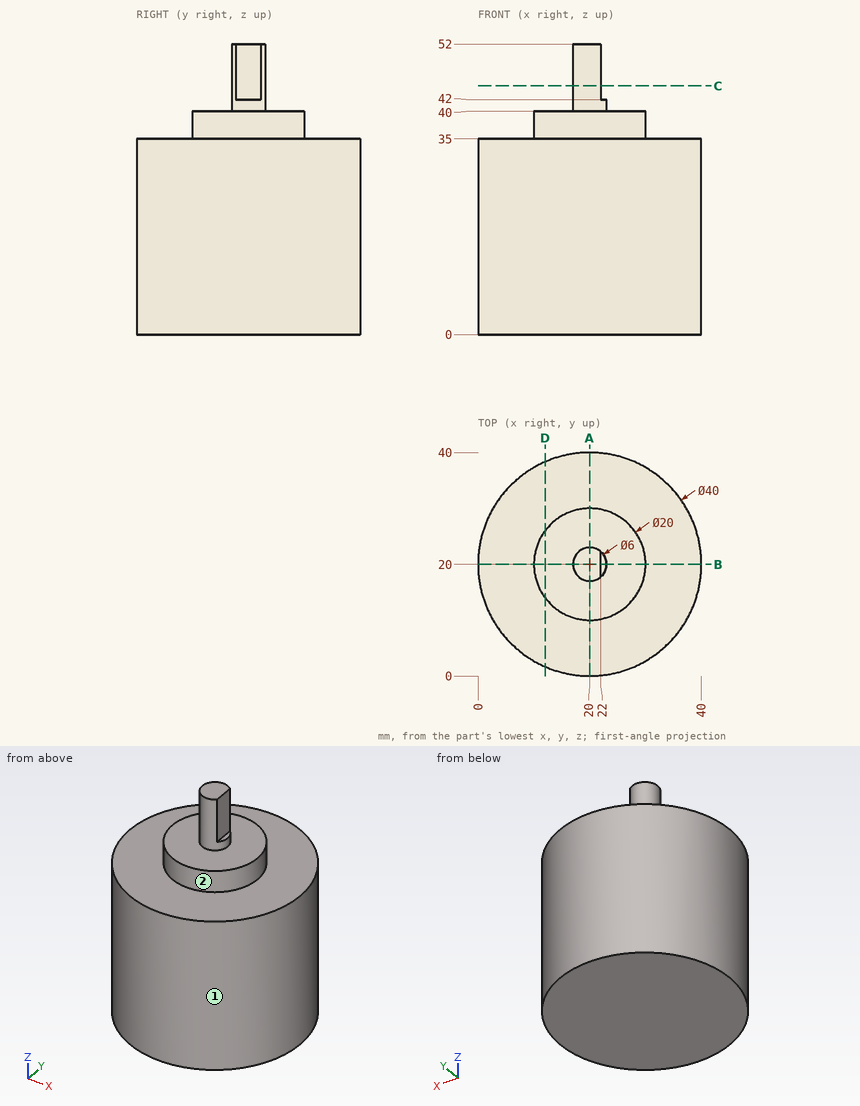
Verification items for this drawing (mm, ordinates from the low corner). A direction names the side the tool comes from. Round coordinates to 2 decimals unless told otherwise and drop trailing zeros. Loops run counter-clockwise (first coordinate to the right, second up) from the corner with the lowest first, then second, coordinate; pieces in that order, holes last. Notation, with made-up numbers: M -6.5,89 L 12.5,89 A18 cw 12.5,113 Z; hole C 73.25,89.5 d9. An arc over 180 degrees is marked long. Answer as a JSON object with one key per item and string values.
1. Section check B-B (y = 20). Record the boundary of the cut face in (x, z), plus the area to 3 significant figures.
Reply:
{"outline": "M 0,0 L 40,0 L 40,35 L 30,35 L 30,40 L 23,40 L 23,42 L 22,42 L 22,52 L 17,52 L 17,40 L 10,40 L 10,35 L 0,35 Z", "area": "1,560 mm²"}
2. Gauge pin test, flat ends, axial feed: P1, Ø10, axis at y = 14.5, z = 29.5, coming from the -X side; P2, Ø0.5, axis at x = 22.5, y = 19, coming from the +Z side; P3, Ø6, axis at x = 17, z = 45.5, coming from the +Y side. Record the tip position at first contact, or that the pin passes through.
Reply:
{"P1": "stops at x = 0.01", "P2": "stops at z = 42", "P3": "stops at y = 23"}
3. Section check A-A (x = 20). Record the boundary of the cut face in (y, z).
Reply:
{"outline": "M 0,0 L 40,0 L 40,35 L 30,35 L 30,40 L 23,40 L 23,52 L 17,52 L 17,40 L 10,40 L 10,35 L 0,35 Z"}
4. Scan lines: line 1 (Z direction, x = 33, y = 28); line 2 (Z direction, x = 20, y = 11.5); line 3 (X direction, y = 34, z = 27). Record each from-to range of solid material in increasing order.
Reply:
{"line 1": "z = 0 to 35", "line 2": "z = 0 to 40", "line 3": "x = 5.72 to 34.28"}
5. Section check D-D (x = 12). Record the boundary of the cut face in (y, z).
Reply:
{"outline": "M 1.67,0 L 38.33,0 L 38.33,35 L 26,35 L 26,40 L 14,40 L 14,35 L 1.67,35 Z"}
6. Section check C-C (z = 44.5). Record the boundary of the cut face in (x, y), plus the area to 3 significant figures.
Reply:
{"outline": "M 22,17.76 L 22,22.24 A3 ccw long Z", "area": "25.2 mm²"}
7. Access from +Z, -Z, +X, -X, +Y, -Y to the whole of each face (thin tool, end or side, straight path). Record for the marked faces 1 and 2.
Reply:
{"face 1": "+Z, -Z", "face 2": "+Z"}
